Build history of the part. All positions in model axes, mm. A direction names the side the tool comes from. Round coordinates to 2 decimals unless told otherwise and drop trailing zeros. Write each loop counter-clockwise with the first axis right and the second up, starting at its lowest first coordinate (ties: lowest second). Pieces come first, ordered by that corner, then holes. Notation, with made-up numbers: M 55,6 L 87,6 A11 ccw 87,19 Z; hole C 5,-1 d7. An arc over 180 degrees is marked long. Write item = value, one per line. Start each with the question number.
Q1. Band-saw the part on B-B on z = 0. Write the cut outline in (x, y), plus the area to 3 significant figures.
Q2. Tool access for faces 1 (the flat face through (3, 2.794, 3)), 2 (the cylindrical face through (1.202, 1.635, 3.816)): list every direction of +Z, -Z, +X, -X, +Y, -Y with a clear straight run to the whole face (end or side of a thin tool).
Q3. Probe L1, parallel to X at y = 1.8, z = 0; L2, parallel to Y at x = 3.25, z = -0.5; L3, parallel to Z at x = -1.75, y = 1.9. List the from-to ranges inside material, lowest first.
Q4. Pull direction X, two halves, no side cores. Call faces 3 (the flat face through (0, 0, 0)), 4 (the flat face through (0, 0.254, 0)), 5 (the cylindrical face through (6.837, 1.18, -0.898)): released by +X, released by -X, zero draft, split by the parting line, or undercut.
Q5. Band-saw the part on A-A on x = 0. Write the cut outline in (y, z), plus the area to 3 significant figures.
Q6. Band-saw the part on C-C on y = 1.65. Write the cut outline in (x, z).
```python
from build123d import *

# Parameters (mm, degrees)
SKETCH1_R           = 6.8961
SKETCH1_R_2         = 4.0005
BOSS_EXTRUDE1_DEPTH = 2.794
SKETCH2_R           = 4.0005
BOSS_EXTRUDE2_DEPTH = 0.254
FILLET1_R           = 0.254
FILLET3_R           = 0.4


with BuildPart() as part:
    # Sketch1 → Boss-Extrude1 (new body)
    with BuildSketch(Plane(origin=(0, 0, 0), x_dir=(1, 0, 0), z_dir=(0, 1, 0))):
        with Locations(Location((0, 0, 0), (0, 0, 270))):
            Circle(SKETCH1_R)
        with Locations(Location((0, 0, 0), (0, 0, 270))):
            Circle(SKETCH1_R_2, mode=Mode.SUBTRACT)
    extrude(amount=BOSS_EXTRUDE1_DEPTH)

    # Sketch2 → Boss-Extrude2 (add)
    with BuildSketch(Plane.XZ):
        with Locations(Location((0, 0, 0), (0, 0, 270))):
            Circle(SKETCH2_R)
    extrude(amount=-BOSS_EXTRUDE2_DEPTH)

    # Fillet1
    fillet1_edges = [part.edges().sort_by_distance(p)[0] for p in [
        (0, 0.254, -4.0005),
    ]]
    fillet(fillet1_edges, radius=FILLET1_R)

    # Fillet3
    fillet3_edges = [part.edges().sort_by_distance(p)[0] for p in [
        (0, 2.794, -6.8961),
    ]]
    fillet(fillet3_edges, radius=FILLET3_R)


solid = part.part
```
Conclusion:
q1.outline = M -6.9,0 L 6.9,0 L 6.9,2.39 A0.4 ccw 6.5,2.79 L 4,2.79 L 4,0.51 A0.25 cw 3.75,0.25 L -3.75,0.25 A0.25 cw -4,0.51 L -4,2.79 L -6.5,2.79 A0.4 ccw -6.9,2.39 Z
q1.area = 18.2 mm^2
q2.face_1 = +Z, -Z, +X, -X, +Y
q2.face_2 = +Y
q3.L1 = -6.9 to -4, 4 to 6.9
q3.L2 = 0 to 0.25
q3.L3 = -6.67 to -3.6, 3.6 to 6.67
q4.face_3 = zero draft
q4.face_4 = undercut
q4.face_5 = split by the parting line
q5.outline = M 0,-6.9 L 2.39,-6.9 A0.4 ccw 2.79,-6.5 L 2.79,-4 L 0.51,-4 A0.25 cw 0.25,-3.75 L 0.25,3.75 A0.25 cw 0.51,4 L 2.79,4 L 2.79,6.5 A0.4 ccw 2.39,6.9 L 0,6.9 Z
q5.area = 18.2 mm^2
q6.outline = C 0,0 d13.79; hole C 0,0 d8
